Could you check a few things on this model? Use its own coordinates, in mm. A direction names the side the tool comes from. Coordinates: 2 decimals unless noted, no trailing zeros. Loops run counter-clockwise (first coordinate to the right, second up) from the corner with the lowest first, then second, coordinate; pieces in that order, holes last. Notation, with made-up numbers: (-24.5, 55.25) - (-8.5, 55.25) arc R22 cw to (-8.5, 90.25) - close; hole circle Ø11 at (61.25, 35.5). An arc over 180 degrees is marked (long way). One line per item, written item: value. Start each with the question number.
(1) On a 3-axis mill with a long thin cutter (end or side, diameter ignored), from which of +Z, -Z, +X, -X, +Y, -Y can I reach the whole of each face in a straight line? I mean faces 1 (the face through (-76.394, 1, 13)), 2 (the face through (-17.624, 0.776, 35.1)). Say none if no direction works.
(2) If we section it at B-B on x = 0: Write out the boundary of the cut face in (y, z).
(3) If we section it at A-A on y = 0: Write out the boundary of the cut face in (x, z), then the cut area to 3 significant figures.
(4) If I drill on line 1 along Z through (x, y) = (45, -13); line 2 along Y through (x, z) = (-6, 27); line 3 along X through (y, z) = (10.5, 26), over which ranges is the centre line in solid material (lowest first)? Write a range as from..to.
(5) If we section it at D-D on y = -40: Write out the boundary of the cut face in (x, z).
(6) I'm going to push flat-ended pins straight in: P1, Ø3, axis at x = -7.5, z = 26, coming from the -Y side; P2, Ø12, axis at x = 55.5, y = -29.5, coming from the +Z side. Where does each tip first touch, or does it pass through?
(7) If we section it at C-C on z = 47: Write out the boundary of the cut face in (x, y).
```python
from build123d import *

# Parameters (mm, degrees)
F2_DEPTH = 25.4
F1_R     = 17.640779
F3_DEPTH = 50.8
F5_DEPTH = 106.248343


with BuildPart() as f2:
    # F0 (on Top) → F2 (new body)
    with BuildSketch(Plane.XY):
        Polygon((-76.394252, 49.22979), (-76.394252, -53.123672), (76.394252, -53.123672), (76.394252, 53.123672), (-76.394252, 53.123672), align=None)
    extrude(amount=F2_DEPTH)

    # F1 (on Top) → F3 (join)
    with BuildSketch(Plane.XY):
        Circle(F1_R)
    extrude(amount=F3_DEPTH)

    # F4 (on face) → F5 (cut, through all)
    with BuildSketch(Plane.XZ.offset(53.123672)):
        Polygon((17.640779, 50.8), (-17.640779, 50.8), (17.640779, 38.1), align=None)
    extrude(amount=-F5_DEPTH, mode=Mode.SUBTRACT)


solid = f2.part
```
Values:
1. face 1: +Z, -Z, -X, +Y, -Y
1. face 2: +Z
2. outline: (-53.12, 0) - (53.12, 0) - (53.12, 25.4) - (17.64, 25.4) - (17.64, 44.45) - (-17.64, 44.45) - (-17.64, 25.4) - (-53.12, 25.4) - close
3. outline: (-76.39, 0) - (76.39, 0) - (76.39, 25.4) - (17.64, 25.4) - (17.64, 38.1) - (-17.64, 50.8) - (-17.64, 25.4) - (-76.39, 25.4) - close
3. area: 4,550 mm2
4. line 1: z = 0..25.4
4. line 2: y = -16.59..16.59
4. line 3: x = -14.18..14.18
5. outline: (-76.39, 0) - (76.39, 0) - (76.39, 25.4) - (-76.39, 25.4) - close
6. P1: stops at y = -53.12
6. P2: stops at z = 25.4
7. outline: (-7.08, -16.16) - (-7.08, 16.16) arc R17.64 ccw to start
